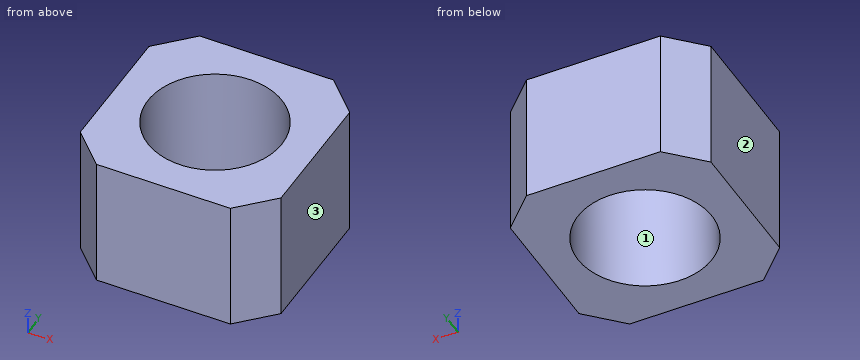
Autodesk Fusion 360 part; units mm, degrees
sketch "Sketch1" plane through (0, 0, 0) normal (0, 0, 1) x (1, 0, 0)
  circle A0 centre (0, 0) radius 4
  line L0 (4, 6) -> (-4, 6)
  line L1 (-6, 4) -> (-6, -4)
  line L2 (-4, -6) -> (4, -6)
  line L3 (6, -4) -> (6, 4)
  line L4 (6, 6) -> (-6, -6) construction
  line L5 (-6, 6) -> (6, -6) construction
  line L6 (4, 6) -> (6, 4)
  line L7 (6, -4) -> (4, -6)
  line L8 (-4, -6) -> (-6, -4)
  line L9 (-4, 6) -> (-6, 4)
  dimension "d1" = 8
  dimension "d2" = 12
  dimension "d3" = 12
  dimension "d4" = 2
  dimension "d5" = 2
  dimension "d6" = 2
  dimension "d7" = 2
  dimension "d8" = 2
  dimension "d9" = 2
  dimension "d10" = 2
  dimension "d11" = 2
extrude "Extrude1" add sketch "Sketch1" along normal blind 8
equation "d5 = d4"
equation "d7 = d6"
equation "d9 = d8"
equation "d11 = d10"
The model under review builds one solid part; all positions refer to its coordinate system, in mm. Face numbers are marked on the shaded views. Round coordinates to 2 decimals unless told otherwise and drop trailing zeros. Loops run counter-clockwise (first coordinate to the right, second up) from the corner with the lowest first, then second, coordinate; pieces in that order, holes last. Notation, with made-up numbers: (10, 49) -> (47, 49) arc R23 cw to (47, 73) -> close; hole circle Ø1 at (67, 21.25). An arc over 180 degrees is marked (long way). Answer as CSV lines item,"result".
1) Add section D-D on x = -4.25. Write out the cut boundary in (y, z).
Geometry results:
outline,"(-5.75, 0) -> (5.75, 0) -> (5.75, 8) -> (-5.75, 8) -> close"
2) Add section A-A on y = 0. Write out the cut boundary in (x, z), plus the area to 3 significant figures.
Geometry results:
outline,"(-6, 0) -> (-4, 0) -> (-4, 8) -> (-6, 8) -> close; (4, 0) -> (6, 0) -> (6, 8) -> (4, 8) -> close"
area,"32.0 mm²"
3) To check wall thickness, follow line 1 along Y through (x, z) = (0, 6); line 2 along Y through (x, z) = (1, 1); line 3 along X through (y, z) = (2, 0.75). State the ranges of each line that lie inside material, in increasing order. Write a range as from..to.
Geometry results:
line 1,"y = -6..-4, 4..6"
line 2,"y = -6..-3.87, 3.87..6"
line 3,"x = -6..-3.46, 3.46..6"
4) For P1, Ø2, axis at x = -0.5, y = -1, coming from the +Z side, flat-tipped, find the tip position at first contact; note if it passes through.
Geometry results:
P1,"passes through"
5) Draft analysis for pull direction X (two halves, no side actions). For the marked faces 1, 2 and 3, state which applies: pulls with the +X half, pulls with the -X half, needs draft (parallel to the pull), parting line crosses it, or undercut.
Geometry results:
face 1,"undercut"
face 2,"pulls with the -X half"
face 3,"pulls with the +X half"
6) Add section C-C on z = 1.75. Write out the cut boundary in (x, y), plus the area to 3 significant figures.
Geometry results:
outline,"(-6, -4) -> (-4, -6) -> (4, -6) -> (6, -4) -> (6, 4) -> (4, 6) -> (-4, 6) -> (-6, 4) -> close; hole circle Ø8 at (0, 0)"
area,"85.7 mm²"
